```python
from build123d import *

# Parameters (mm, degrees)
CYLINDER001_R     = 24.5
CYLINDER001_DEPTH = 2
SKETCH_R          = 23
SKETCH_R_2        = 22
PAD_DEPTH         = 10
SKETCH002_R       = 1.5
SKETCH002_R_2     = 4
POCKET001_DEPTH   = 10


with BuildPart() as part:
    # Cylinder001 → Cylinder001 (new body)
    with BuildSketch(Plane.XY):
        Circle(CYLINDER001_R)
    extrude(amount=CYLINDER001_DEPTH)

    # Sketch → Pad (new body)
    with BuildSketch(Plane.XY.offset(2)):
        Circle(SKETCH_R)
        Circle(SKETCH_R_2, mode=Mode.SUBTRACT)
    extrude(amount=PAD_DEPTH)

    # Sketch002 → Pocket001 (cut)
    with BuildSketch(Plane.XY.offset(2)):
        with Locations((-18.5, 0)):
            Circle(SKETCH002_R)
        with Locations((18.5, 0)):
            Circle(SKETCH002_R)
        with Locations((0, -16)):
            Circle(SKETCH002_R_2)
    extrude(amount=-POCKET001_DEPTH, mode=Mode.SUBTRACT)


solid = part.part
```
Check sheet for the modelled part. Datum: model origin and axes. Units: mm. A direction names the side the tool comes from. Give positions to 0.01 mm unless a question says otherwise; leave off trailing zeros. Loops run counter-clockwise (first coordinate to the right, second up) from the corner with the lowest first, then second, coordinate; pieces in that order, holes last. Notation, with made-up numbers: M 75,15 L 79,15 A20 ccw 79,37 Z; hole C 10.5,-28 d4. An arc over 180 degrees is marked long. Answer as CSV lines item,"result".
Item 1: Set-up check for faces 4 (the face through (-4.769, -21.477, 6.93)), 5 (the face through (13.17, 20.66, 0.99)): record each of +Z, -Z, +X, -X, +Y, -Y from which the full face is reachable in a straight line by a thin tool's end or side.
Reply:
face 4,"+Z"
face 5,"+Z, -Z"
Item 2: Sectioned sample at B-B, the plane y = 0. Enter the section's corners in (x, z), then the cut area to 3 significant figures.
Reply:
outline,"M -24.5,0 L -20,0 L -20,2 L -22,2 L -22,12 L -23,12 L -23,2 L -24.5,2 Z; M -17,0 L 17,0 L 17,2 L -17,2 Z; M 20,0 L 24.5,0 L 24.5,2 L 23,2 L 23,12 L 22,12 L 22,2 L 20,2 Z"
area,"106 mm^2"
Item 3: Sectioned sample at A-A, the plane x = 0. Enter the section's corners in (y, z), then the cut area to 3 significant figures.
Reply:
outline,"M -24.5,0 L -20,0 L -20,2 L -22,2 L -22,12 L -23,12 L -23,2 L -24.5,2 Z; M -12,0 L 24.5,0 L 24.5,2 L 23,2 L 23,12 L 22,12 L 22,2 L -12,2 Z"
area,"102 mm^2"
Item 4: Scan lines: L1, parallel to Y at x = 0, z = 7.5; L2, parallel to Z at x = -7, y = 12; L3, parallel to X at y = -1, z = 4.25. Record each from-to range of solid material in increasing order.
Reply:
L1,"-23 to -22, 22 to 23"
L2,"0 to 2"
L3,"-22.98 to -21.98, 21.98 to 22.98"
Item 5: Depth check by flat-ended pin: pin 1 Ø1 at (y, z) = (-12, 5.5) entering from +X; pin 2 Ø2 at (x, z) = (13.5, 9) entering from +Y; pin 3 Ø4 at (x, z) = (12, 5.5) entering from -Y. Enter the tip coordinate at first touch or a pass-through.
Reply:
pin 1,"x = 19.92"
pin 2,"y = 19.31"
pin 3,"y = -20.71"
Item 6: Draft check along Y on faces 1 (the face through (-20, 0, 1)), 2 (the face through (0, 0, 0)), 3 (the face through (-2.994, 22.804, 6.93)). Enter one of: pulls with the +Y half, pulls with the -Y half, needs draft (parallel to the pull), parting line crosses it, or undercut.
Reply:
face 1,"undercut"
face 2,"needs draft"
face 3,"parting line crosses it"
Item 7: Sectioned sample at D-D, the plane z = 7.25. Enter the section's corners in (x, y).
Reply:
outline,"C 0,0 d46; hole C 0,0 d44"
Item 8: Sectioned sample at C-C, the plane y = -16. Enter the section's corners in (x, z), then the cut area to 3 significant figures.
Reply:
outline,"M -18.55,0 L -4,0 L -4,2 L -15.1,2 L -15.1,12 L -16.52,12 L -16.52,2 L -18.55,2 Z; M 4,0 L 18.55,0 L 18.55,2 L 16.52,2 L 16.52,12 L 15.1,12 L 15.1,2 L 4,2 Z"
area,"86.7 mm^2"
